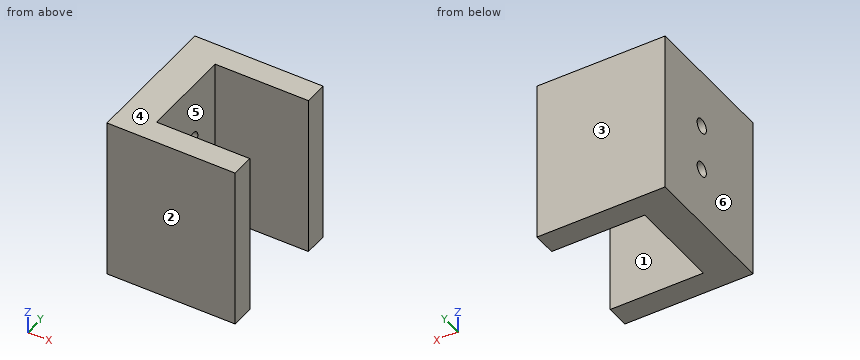
from build123d import *

# Parameters (mm, degrees)
SKETCH1_W           = 4.7625
SKETCH1_H           = 22.225
BOSS_EXTRUDE1_DEPTH = 3.175
SKETCH2_W           = 4.7625
SKETCH2_H           = 22.225
BOSS_EXTRUDE2_DEPTH = 15.875
SKETCH3_R           = 1
CUT_EXTRUDE1_DEPTH  = 5.7625
SKETCH5_W           = 22.225
SKETCH5_H           = 3.175
BOSS_EXTRUDE3_DEPTH = 12.7


with BuildPart() as part:
    # Sketch1 → Boss-Extrude1 (new body)
    with BuildSketch(Plane(origin=(0, 0, 0), x_dir=(1, 0, 0), z_dir=(0, 1, 0))):
        Rectangle(SKETCH1_W, SKETCH1_H)
    extrude(amount=BOSS_EXTRUDE1_DEPTH)

    # Sketch2 → Boss-Extrude2 (add)
    with BuildSketch(Plane(origin=(0, 3.175, 0), x_dir=(1, 0, 0), z_dir=(0, 1, 0))):
        Rectangle(SKETCH2_W, SKETCH2_H)
    extrude(amount=BOSS_EXTRUDE2_DEPTH)

    # Sketch3 → Cut-Extrude1 (cut, through all)
    with BuildSketch(Plane.ZY.offset(2.38125)):
        with Locations((3.175, 11.1125)):
            Circle(SKETCH3_R)
        with Locations((-3.175, 11.1125)):
            Circle(SKETCH3_R)
    extrude(amount=-CUT_EXTRUDE1_DEPTH, mode=Mode.SUBTRACT)

    # Sketch5 → Boss-Extrude3 (add)
    with BuildSketch(Plane(origin=(2.38125, 0, 0), x_dir=(0, 0, -1), z_dir=(1, 0, 0))):
        with Locations((0, 17.4625)):
            Rectangle(SKETCH5_W, SKETCH5_H)
        with Locations((0, 1.5875)):
            Rectangle(SKETCH5_W, SKETCH5_H)
    extrude(amount=BOSS_EXTRUDE3_DEPTH)


solid = part.part
Can you work these out from the model? Positions are in its coordinate system, mm. Face numbers are marked on the shaded views. A direction names the side the tool comes from. Coordinates: 2 decimals unless noted, no trailing zeros. Order: outer loops, then holes, each group sorted by start corner. A loop starts at its lowest first (then second) coordinate and runs counter-clockwise, first axis right, second up. Notation, with made-up numbers: M 36,67 L 72,67 A34 cw 72,97 Z; hole C 26,-0.5 d3. An arc over 180 degrees is marked long. Write item = value, one per line.
(1) Suppose I cut it at B-B on z = 3.5. Please give me the cut outline in (x, y) (3 decimals), plus the area to 3 significant figures.
Results are:
outline = M -2.381,0 L 15.081,0 L 15.081,3.175 L 2.381,3.175 L 2.381,10.167 L -2.381,10.167 Z; M -2.381,12.058 L 2.381,12.058 L 2.381,15.875 L 15.081,15.875 L 15.081,19.05 L -2.381,19.05 Z
area = 162 mm2
(2) I need wall thicknesses on line 1 along Y through (x, z) = (9, 8.5) (3 decimals); line 2 along X through (y, z) = (6, 6); line 3 along Z through (x, y) = (2, 10.5). Which ranges of each line are inside material? Lowest first, please. Write a range as [from, to].
Results are:
line_1 = [0, 3.175], [15.875, 19.05]
line_2 = [-2.38, 2.38]
line_3 = [-11.11, -3.97], [-2.38, 2.38], [3.97, 11.11]
(3) If we mould it in two halves opening along Y, with no side actions, what happens to the marked faces 1, 2, 3 and 4? For each: pulls with the +Y half, pulls with the -Y half, needs draft (parallel to the pull), parting line crosses it, or undercut.
Results are:
face_1 = undercut
face_2 = pulls with the -Y half
face_3 = pulls with the +Y half
face_4 = needs draft
(4) Suppose I cut it at C-C on y = 10.5. Please give me the cut outline in (x, z), plus the area to 3 significant figures.
Results are:
outline = M -2.38,-11.11 L 2.38,-11.11 L 2.38,-3.97 L -2.38,-3.97 Z; M -2.38,-2.38 L 2.38,-2.38 L 2.38,2.38 L -2.38,2.38 Z; M -2.38,3.97 L 2.38,3.97 L 2.38,11.11 L -2.38,11.11 Z
area = 90.8 mm2
(5) Suppose I cut it at D-D on z = -4.5. Please give me the cut outline in (x, y) (3 decimals), plus the area to 3 significant figures.
Results are:
outline = M -2.381,0 L 15.081,0 L 15.081,3.175 L 2.381,3.175 L 2.381,15.875 L 15.081,15.875 L 15.081,19.05 L -2.381,19.05 Z
area = 171 mm2
(6) For the marked faces 5 and 6, which set-ups out of +Z, -Z, +X, -X, +Y, -Y let a thin tool reach every point of the face, with its end or its side?
Results are:
face_5 = +Z, -Z, +X
face_6 = +Z, -Z, -X, +Y, -Y
